```python
from build123d import *

# Parameters (mm, degrees)
SKETCH1_W           = 25.4
SKETCH1_H           = 12.7
BOSS_EXTRUDE1_DEPTH = 3.175
CUT_EXTRUDE1_DEPTH  = 3.175
SKETCH3_W           = 25.4
SKETCH3_H           = 3.175
BOSS_EXTRUDE2_DEPTH = 61.341
SKETCH4_W           = 25.4
SKETCH4_H           = 1.905
BOSS_EXTRUDE3_DEPTH = 1.27


with BuildPart() as part:
    # Sketch1 → Boss-Extrude1 (new body)
    with BuildSketch(Plane.XY):
        with Locations((4.390957447, -0.776861702)):
            Rectangle(SKETCH1_W, SKETCH1_H)
    extrude(amount=BOSS_EXTRUDE1_DEPTH)

    # Sketch2 → Cut-Extrude1 (cut)
    with BuildSketch(Plane.XY.offset(3.175)):
        with BuildLine():
            ThreePointArc((12.468157447, 2.398138298), (11.962272279, 3.61945313), (10.740957447, 4.125338298))
            Line((10.740957447, 4.125338298), (10.740957447, 0.670938298))
            ThreePointArc((10.740957447, 0.670938298), (11.962272279, 1.176823465), (12.468157447, 2.398138298))
        make_face()
        with BuildLine():
            Line((10.740957447, 0.670938298), (10.740957447, 4.125338298))
            ThreePointArc((10.740957447, 4.125338298), (9.013757447, 2.398138298), (10.740957447, 0.670938298))
        make_face()
        with BuildLine():
            ThreePointArc((-0.231842553, 2.398138298), (-0.737727721, 3.61945313), (-1.959042553, 4.125338298))
            Line((-1.959042553, 4.125338298), (-1.959042553, 0.670938298))
            ThreePointArc((-1.959042553, 0.670938298), (-0.737727721, 1.176823465), (-0.231842553, 2.398138298))
        make_face()
        with BuildLine():
            Line((-1.959042553, 0.670938298), (-1.959042553, 4.125338298))
            ThreePointArc((-1.959042553, 4.125338298), (-3.686242553, 2.398138298), (-1.959042553, 0.670938298))
        make_face()
    extrude(amount=-CUT_EXTRUDE1_DEPTH, mode=Mode.SUBTRACT)

    # Sketch3 → Boss-Extrude2 (add)
    with BuildSketch(Plane.XY.offset(3.175)):
        with Locations((4.390957447, -5.539361702)):
            Rectangle(SKETCH3_W, SKETCH3_H)
    extrude(amount=BOSS_EXTRUDE2_DEPTH)

    # Sketch4 → Boss-Extrude3 (add)
    with BuildSketch(Plane.XZ.offset(7.126861702)):
        with Locations((4.390957447, 63.5635)):
            Rectangle(SKETCH4_W, SKETCH4_H)
    extrude(amount=BOSS_EXTRUDE3_DEPTH)


solid = part.part
```
CAD build for the part. Positions are in the model's coordinates, mm. A direction names the side the tool comes from. Round coordinates to 2 decimals unless told otherwise and drop trailing zeros. Write each loop counter-clockwise with the first axis right and the second up, starting at its lowest first coordinate (ties: lowest second). Pieces come first, ordered by that corner, then holes.
Item 1: Band-saw the part on A-A on x = 5. Write the cut outline in (y, z) (3 decimals).
Filled in:
outline: (-8.397, 62.611) - (-7.127, 62.611) - (-7.127, 0) - (5.573, 0) - (5.573, 3.175) - (-3.952, 3.175) - (-3.952, 64.516) - (-8.397, 64.516) - close
Item 2: Tool access for faces 1 (the flat face through (4, 5.573, 2)), 2 (the flat face through (4, 1, 3.175)), 3 (the flat face through (4, -8, 62.611)): list every direction of +Z, -Z, +X, -X, +Y, -Y with a clear straight run to the whole face (end or side of a thin tool).
Filled in:
face 1: +Z, -Z, +X, -X, +Y
face 2: +Z, +X, -X, +Y
face 3: -Z, +X, -X, -Y
Item 3: Band-saw the part on C-C on z = 44. Write the cut outline in (x, y).
Filled in:
outline: (-8.31, -7.13) - (17.09, -7.13) - (17.09, -3.95) - (-8.31, -3.95) - close
Item 4: Drop flat-ended pins along their axis: pin 1 Ø12 at (x, z) = (11.5, 56) entering from +Y; pin 2 Ø10 at (x, z) = (0.5, 31.5) entering from -Y; pin 3 Ø5 at (x, y) = (-1, 4) entering from +Z (3 decimals). Give the stop position or say it passes through.
Filled in:
pin 1: stops at y = -3.95
pin 2: stops at y = -7.13
pin 3: stops at z = 3.175
Item 5: Band-saw the part on B-B on y = -3. Write the cut outline in (x, z) (3 decimals).
Filled in:
outline: (-8.309, 0) - (17.091, 0) - (17.091, 3.175) - (-8.309, 3.175) - close
Item 6: Drill centre lines: L1, parallel to Y at x = 12, z = 52.5; L2, parallel to Z at x = -5, y = -0.75 (3 decimals); L3, parallel to Z at x = 7.5, y = -7.5. Where is each one in solid material? Low to high.
Filled in:
L1: y = -7.13 to -3.95
L2: z = 0 to 3.175
L3: z = 62.61 to 64.52
